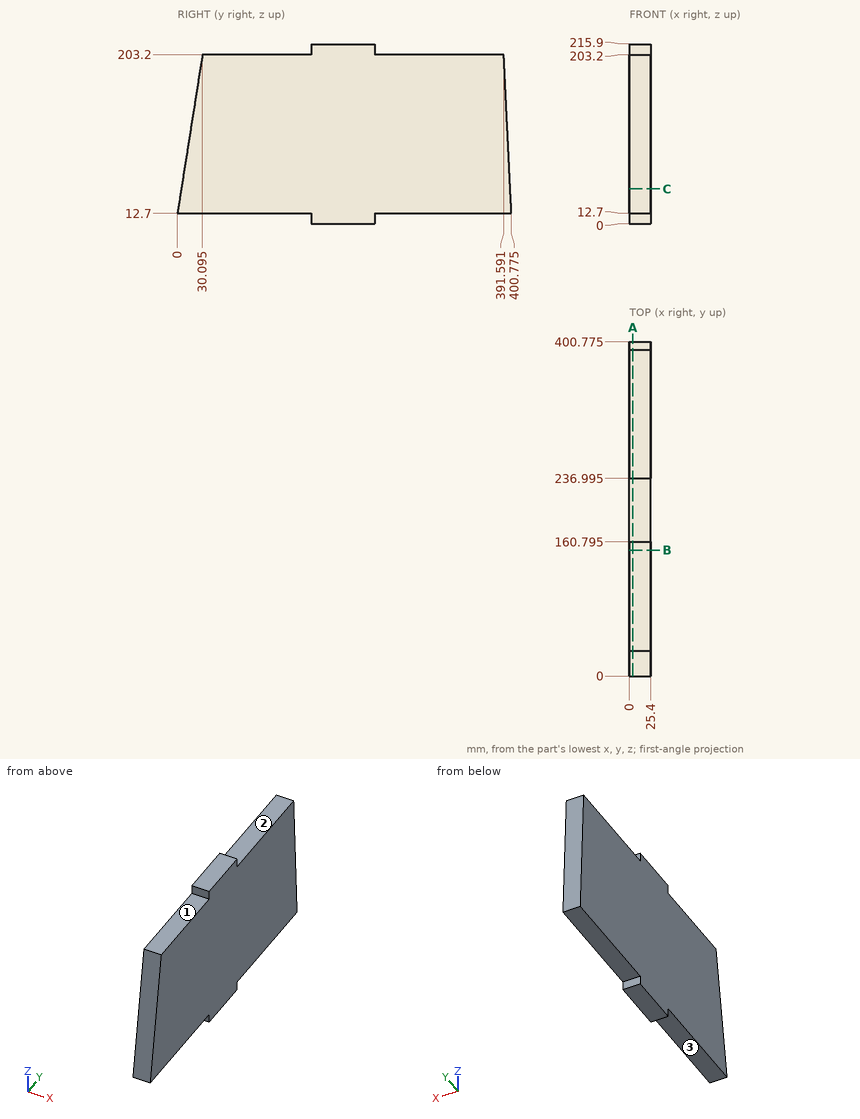
Check sheet for the drawn part. Datum: minimum x, y, z corner. Units: mm. A direction names the side the tool comes from. Give positions to 0.01 mm unless a question says otherwise; leave off trailing zeros. Order: outer loops, then holes, each group sorted by start corner. A loop starts at its lowest first (then second) coordinate and runs counter-clockwise, first axis right, second up. Notation, with made-up numbers: (-10.5, 24.5) -> (27.5, 24.5) arc R27 cw to (27.5, 54.5) -> close; hole circle Ø7 at (86, -21.5). An arc over 180 degrees is marked (long way). Return JSON: item names as keys, results as strings.
1. Cross-section at C-C, the plane z = 42. Record the cut outline in (x, y).
From the geometry:
{"outline": "(0, 4.63) -> (25.4, 4.63) -> (25.4, 399.36) -> (0, 399.36) -> close"}
2. Set-up check for the marked faces 1, 2 and 3: record each of +Z, -Z, +X, -X, +Y, -Y from which the full face is reachable in a straight line by a thin tool's end or side.
From the geometry:
{"face 1": "+Z, +X, -X, -Y", "face 2": "+Z, +X, -X, +Y", "face 3": "-Z, +X, -X, -Y"}
3. Material ranges on probe 1 along Z at (x, y) = (23.5, 138.5); probe 2 along Y at (x, z) = (3, 32.5); probe 3 along Y at (x, z) = (13, 23.5) (1 decimal), recorded low to high. Write a range as [from, to].
From the geometry:
{"probe 1": "[12.7, 203.2]", "probe 2": "[3.13, 399.82]", "probe 3": "[1.7, 400.3]"}
4. Go/stop test with flat-tipped pins: P1, Ø2, axis at x = 17, y = 289, coming from the -Z side; P2, Ø7.5, axis at x = 11, y = 295, coming from the +Z side; P3, Ø10, axis at x = 16, z = 41.5, coming from the +Y side. Record where each tip stops, or that it passes through.
From the geometry:
{"P1": "z = 12.7", "P2": "z = 203.2", "P3": "y = 399.63"}
5. Cross-section at B-B, the plane y = 151. Record the cut outline in (x, z).
From the geometry:
{"outline": "(0, 12.7) -> (25.4, 12.7) -> (25.4, 203.2) -> (0, 203.2) -> close"}
6. Cross-section at A-A, the plane x = 4. Record the cut outline in (y, z) (1 decimal).
From the geometry:
{"outline": "(0, 12.7) -> (160.8, 12.7) -> (160.8, 0) -> (237, 0) -> (237, 12.7) -> (400.8, 12.7) -> (391.6, 203.2) -> (237, 203.2) -> (237, 215.9) -> (160.8, 215.9) -> (160.8, 203.2) -> (30.1, 203.2) -> close"}
